The listing builds one solid part. Answer for the finished solid, in the listing's coordinates (mm). A direction names the side the tool comes from. Coordinates: 2 decimals unless noted, no trailing zeros. Loops run counter-clockwise (first coordinate to the right, second up) from the corner with the lowest first, then second, coordinate; pieces in that order, holes last. Notation, with made-up numbers: (-20, 7.5) - (35, 7.5) arc R18 ccw to (35, 42.5) - close; hole circle Ø10 at (-13, 74). An arc over 180 degrees is marked (long way). One line per question, with ' | ' between items.
from build123d import *

# Parameters (mm, degrees)
F1_DEPTH = 63.5
F2_DEPTH = 25.4
F3_DEPTH = 7.9375
F5_R     = 6.35


with BuildPart() as f1:
    # F0 (on Front) → F1 (new body, symmetric)
    with BuildSketch(Plane.XZ):
        Polygon((-41.275, 9.525), (-41.275, -9.525), (41.275, -9.525), (41.275, 9.525), (22.225, 9.525), align=None)
    extrude(amount=F1_DEPTH, both=True)

    # F0 (on Front) → F2 (join, symmetric)
    with BuildSketch(Plane.XZ):
        with BuildLine():
            Line((22.225, 9.525), (41.275, 9.525))
            Line((41.275, 9.525), (41.275, 27.0002))
            ThreePointArc((41.275, 27.0002), (45.9246798487, 38.2255201513), (57.15, 42.8752))
            Line((57.15, 42.8752), (60.325, 42.8752))
            Line((60.325, 42.8752), (60.325, 61.9252))
            Line((60.325, 61.9252), (57.15, 61.9252))
            add(Edge.make_bspline(
                [(55.8342690967, 61.900407409), (56.274218932, 61.9111436169), (56.7128210879, 61.9194148517), (57.15, 61.9252)],
                knots=[110.352429098, 110.352429098, 110.352429098, 110.352429098, 111.5045361635, 111.5045361635, 111.5045361635, 111.5045361635], degree=3))
            ThreePointArc((55.8342690967, 61.900407409), (31.9934151086, 51.2262574919), (22.225, 27.0002))
            Line((22.225, 27.0002), (22.225, 9.525))
        make_face()
        Polygon((60.325, 66.675), (60.325, 61.9252), (60.325, 42.8752), (60.325, 38.1), (85.725, 38.1), (85.576608777, 66.675), align=None)
    extrude(amount=F2_DEPTH, both=True)

    # F0 (on Front) → F3 (join, symmetric)
    with BuildSketch(Plane.XZ):
        with BuildLine():
            add(Edge.make_bspline(
                [(-41.275, 9.525), (-40.8094440998, 37.2290406247), (13.6944936723, 60.8720597372), (55.8342690967, 61.900407409)],
                knots=[0, 0, 0, 0, 110.352429098, 110.352429098, 110.352429098, 110.352429098], degree=3))
            Line((-41.275, 9.525), (22.225, 9.525))
            Line((22.225, 9.525), (22.225, 27.0002))
            ThreePointArc((22.225, 27.0002), (31.9934151086, 51.2262574919), (55.8342690967, 61.900407409))
        make_face()
    extrude(amount=F3_DEPTH, both=True)

    # F0 (on Front) → F4 (revolve)
    with BuildSketch(Plane.XZ):
        Polygon((111.125, 66.675), (85.576608777, 66.675), (85.725, 38.1), (111.125, 38.1), align=None)
    revolve(axis=Axis((85.6508043885, 0, 52.3875), (-0.0051929737, 0, 0.9999865164)))

    # F5
    f5_edges = [f1.edges().sort_by_distance(p)[0] for p in [
        (-41.275, -63.5, 0),
        (41.275, -63.5, 0),
        (41.275, 63.5, 0),
        (-41.275, 63.5, 0),
    ]]
    fillet(f5_edges, radius=F5_R)


solid = f1.part
Item 1: Find section B-B, the plane y = 44. Write down the section's boundary in (x, z) (3 decimals).
Taken from the geometry:
outline: (-41.275, -9.525) - (41.275, -9.525) - (41.275, 9.525) - (-41.275, 9.525) - close
Item 2: Which of the six approach directions +Z, -Z, +X, -X, +Y, -Y give full straight-line access (tool end or side, diameter ignored) to faces 1 (the face through (22.225, -17, 18)), 2 (the face through (41.275, -1, 4))?
Taken from the geometry:
face 1: +Z, -X, -Y | face 2: -Z, +X, +Y, -Y
Item 3: Find section A-A, the plane z = -1. Write down the section's boundary in (x, y) (3 decimals), plus the area to 3 significant figures.
Taken from the geometry:
outline: (-41.275, -57.15) arc R6.35 ccw to (-34.925, -63.5) - (34.925, -63.5) arc R6.35 ccw to (41.275, -57.15) - (41.275, 57.15) arc R6.35 ccw to (34.925, 63.5) - (-34.925, 63.5) arc R6.35 ccw to (-41.275, 57.15) - close | area: 10,400 mm2
Item 4: The mould has two halves that part along X. Classify faces 3 (the face through (45.8, -0.4, 38.1)), 4 (the face through (39.365, 61.689, 0.133)), 5 (the face through (53, -25.4, 45)): pulls with the +X half, pulls with the -X half, needs draft (parallel to the pull), parting line crosses it, or undercut.
Taken from the geometry:
face 3: undercut | face 4: pulls with the +X half | face 5: needs draft
Item 5: Each of these flat-tipped pins is pushed along its axis until it touches: pin 1 Ø5 at (y, z) = (-15, 16.5) entering from -X (3 decimals); pin 2 Ø1 at (y, z) = (-23, 29) entering from -X; pin 3 Ø1 at (x, y) = (58, 7.5) entering from +Z. Where does it stop, or does it pass through?
Taken from the geometry:
pin 1: stops at x = 22.225 | pin 2: stops at x = 22.26 | pin 3: stops at z = 61.93
Item 6: Find the intervals of material crossed by line 1 (Y direction, x = 14.5, z = 21); line 2 (Z direction, x = -14, y = 14) (3 decimals); line 3 (X direction, y = 53, z = -0.5) (3 decimals), in increasing order. Write a range as [from, to].
Taken from the geometry:
line 1: y = [-7.94, 7.94] | line 2: z = [-9.525, 9.525] | line 3: x = [-41.275, 41.275]
